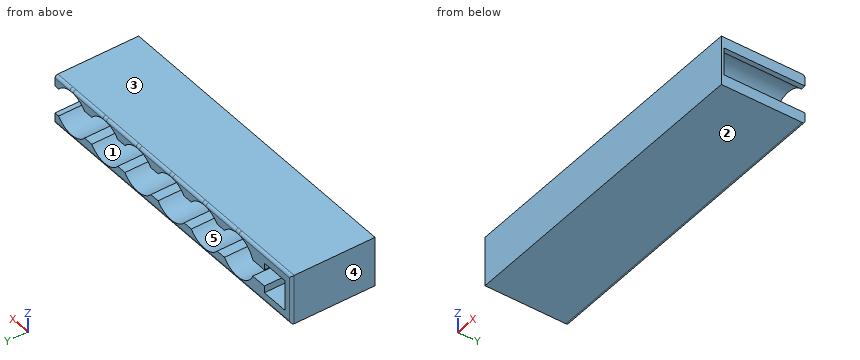
```python
from build123d import *

# Parameters (mm, degrees)
SKETCH1_W           = 114
SKETCH1_H           = 18
BOSS_EXTRUDE1_DEPTH = 30
CUT_EXTRUDE2_DEPTH  = 29
SKETCH4_W           = 6
SKETCH4_H           = 6
CUT_EXTRUDE4_DEPTH  = 29
FILLET1_R           = 1
SKETCH5_W           = 10
SKETCH5_H           = 11
CUT_EXTRUDE6_DEPTH  = 29


with BuildPart() as part:
    # Sketch1 → Boss-Extrude1 (new body)
    with BuildSketch(Plane(origin=(0, 0, 0), x_dir=(1, 0, 0), z_dir=(0, 1, 0))):
        Rectangle(SKETCH1_W, SKETCH1_H)
    extrude(amount=BOSS_EXTRUDE1_DEPTH)

    # Sketch2 → Cut-Extrude2 (cut)
    with BuildSketch(Plane(origin=(0, 30, 0), x_dir=(1, 0, 0), z_dir=(0, 1, 0))):
        with BuildLine():
            Line((-21.244998569, 4.958042294), (-24.755000861, 4.958042294))
            ThreePointArc((-24.755000861, 4.958042294), (-39, -0.041954456), (-24.755003142, -5.041957706))
            Line((-24.755003142, -5.041957706), (-21.244997428, -5.041957706))
            ThreePointArc((-21.244997428, -5.041957706), (-15, -8.041956993), (-8.755002572, -5.041957706))
            Line((-8.755002572, -5.041957706), (-5.244997998, -5.041957706))
            ThreePointArc((-5.244997998, -5.041957706), (1, -8.041957706), (7.244997998, -5.041957706))
            Line((7.244997998, -5.041957706), (10.755002002, -5.041957706))
            ThreePointArc((10.755002002, -5.041957706), (17, -8.041957706), (23.244997998, -5.041957706))
            Line((23.244997998, -5.041957706), (26.755002002, -5.041957706))
            ThreePointArc((26.755002002, -5.041957706), (33, -8.041957706), (39.244997998, -5.041957706))
            Line((39.244997998, -5.041957706), (42.755002002, -5.041957706))
            ThreePointArc((42.755002002, -5.041957706), (49, -8.041957706), (55.244997998, -5.041957706))
            Line((55.244997998, -5.041957706), (57, -5.041957706))
            Line((57, -5.041957706), (57, 4.958042294))
            Line((57, 4.958042294), (55.244997998, 4.958042294))
            ThreePointArc((55.244997998, 4.958042294), (49, 7.958042294), (42.755002002, 4.958042294))
            Line((42.755002002, 4.958042294), (39.244997998, 4.958042294))
            ThreePointArc((39.244997998, 4.958042294), (33, 7.958042294), (26.755002002, 4.958042294))
            Line((26.755002002, 4.958042294), (23.244997998, 4.958042294))
            ThreePointArc((23.244997998, 4.958042294), (17, 7.958042294), (10.755002002, 4.958042294))
            Line((10.755002002, 4.958042294), (7.244997998, 4.958042294))
            ThreePointArc((7.244997998, 4.958042294), (1, 7.958042294), (-5.244997998, 4.958042294))
            Line((-5.244997998, 4.958042294), (-8.755001431, 4.958042294))
            ThreePointArc((-8.755001431, 4.958042294), (-15, 7.958043007), (-21.244998569, 4.958042294))
        make_face()
    extrude(amount=-CUT_EXTRUDE2_DEPTH, mode=Mode.SUBTRACT)

    # Sketch4 → Cut-Extrude4 (cut)
    with BuildSketch(Plane(origin=(0, 30, 0), x_dir=(1, 0, 0), z_dir=(0, 1, 0))):
        with Locations((-41, 0)):
            Rectangle(SKETCH4_W, SKETCH4_H)
    extrude(amount=-CUT_EXTRUDE4_DEPTH, mode=Mode.SUBTRACT)

    # Fillet1
    fillet1_edges = [part.edges().sort_by_distance(p)[0] for p in [
        (-57, 30, 0),
        (0, 30, 9),
        (0, 30, -9),
    ]]
    fillet(fillet1_edges, radius=FILLET1_R)

    # Sketch5 → Cut-Extrude6 (cut)
    with BuildSketch(Plane(origin=(0, 30, 0), x_dir=(1, 0, 0), z_dir=(0, 1, 0))):
        with Locations((-49, 0)):
            Rectangle(SKETCH5_W, SKETCH5_H)
    extrude(amount=-CUT_EXTRUDE6_DEPTH, mode=Mode.SUBTRACT)


solid = part.part
```
Source: CAD feature listing. Evaluate the final solid. Frame: model axes, mm. Face numbers are marked on the shaded views. A direction names the side the tool comes from. Give positions to 0.01 mm unless a question says otherwise; leave off trailing zeros. Write each loop counter-clockwise with the first axis right and the second up, starting at its lowest first coordinate (ties: lowest second). Pieces come first, ordered by that corner, then holes.
1. Section query C-C (x = -45). Return the cut outline in (y, z), then the cut area to 3 significant figures.
2. Pull-direction query (Z, two-part tool) for the marked faces 3, 4 and 5; classes: +Z half, -Z half, draft (parallel to the pull), parting line (faces both ways), or undercut.
3. Material intervals for line 1 along Z through (x, y) = (-24, 23); line 2 along Y through (x, z) = (33, -1.25); line 3 along X through (y, z) = (20.5, -2.25), sorted ascending.
4. First-contact query: pin 1 (3.5 mm diameter, centred on y = 19, z = 1.5, fed in from +X); pin 2 (1 mm diameter, centred on y = 13, z = 4, fed in from +X). Flat tips, straight axial feed; report the tip coordinate or a pass-through.
5. Section query B-B (z = -0.25). Return the cut outline in (x, y), then the cut area to 3 significant figures.
6. Section query A-A (x = 41). Return the cut outline in (y, z), then the cut area to 3 significant figures.
7. Access query for the marked faces 1 and 2. Directions: +Z, -Z, +X, -X, +Y, -Y. A direction counts if a zero-diameter tool reaches every point of the face in a straight line with its end or side. Return the directions, or none.
Output values:
1. outline: (0, -9) - (29, -9) arc R1 ccw to (30, -8) - (30, -5.5) - (1, -5.5) - (1, 5.5) - (30, 5.5) - (30, 8) arc R1 ccw to (29, 9) - (0, 9) - close
1. area: 221 mm2
2. face 3: +Z half
2. face 4: draft
2. face 5: undercut
3. line 1: z = -9 to -4.96, 5.04 to 9
3. line 2: y = 0 to 1
3. line 3: x = -57 to -54
4. pin 1: stops at x = -38.33
4. pin 2: stops at x = -37.64
5. outline: (-57, 0) - (57, 0) - (57, 1) - (-54, 1) - (-54, 30) - (-56, 30) arc R1 ccw to (-57, 29) - close
5. area: 201 mm2
6. outline: (0, -9) - (29, -9) arc R1 ccw to (30, -8) - (30, -4.96) - (1, -4.96) - (1, 5.04) - (30, 5.04) - (30, 8) arc R1 ccw to (29, 9) - (0, 9) - close
6. area: 250 mm2
7. face 1: +Y
7. face 2: -Z, +X, -X, +Y, -Y
